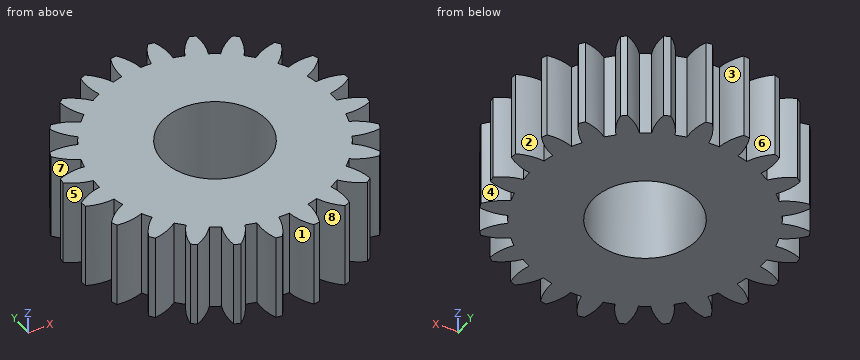
```python
from build123d import *

# Parameters (mm, degrees)
SKETCH2_R           = 3.81
BOSS_EXTRUDE1_DEPTH = 6.35


with BuildPart() as part:
    # Sketch2 → Boss-Extrude1 (new body)
    with BuildSketch(Plane.XY):
        with BuildLine():
            ThreePointArc((-42.015017319, -22.945367918), (-41.531469039, -22.120633406), (-41.268457962, -21.20148645))
            ThreePointArc((-41.268457962, -21.20148645), (-40.889005651, -21.209938725), (-40.50955334, -21.20148645))
            ThreePointArc((-40.50955334, -21.20148645), (-40.246542262, -22.120633406), (-39.762993983, -22.945367918))
            ThreePointArc((-39.762993983, -22.945367918), (-39.542138505, -22.918710388), (-39.321909019, -22.887297981))
            ThreePointArc((-39.321909019, -22.887297981), (-39.068294246, -21.965514112), (-39.052137791, -21.009614053))
            ThreePointArc((-39.052137791, -21.009614053), (-38.683427394, -20.919568839), (-38.319092217, -20.813195084))
            ThreePointArc((-38.319092217, -20.813195084), (-37.827150287, -21.632950591), (-37.146621516, -22.304431452))
            ThreePointArc((-37.146621516, -22.304431452), (-36.940190983, -22.221520651), (-36.735595764, -22.13417901))
            ThreePointArc((-36.735595764, -22.13417901), (-36.729197926, -21.178163832), (-36.960997129, -20.250653679))
            ThreePointArc((-36.960997129, -20.250653679), (-36.628155651, -20.068247408), (-36.303766447, -19.871201369))
            ThreePointArc((-36.303766447, -19.871201369), (-35.616418695, -20.535700443), (-34.785286345, -21.008167342))
            ThreePointArc((-34.785286345, -21.008167342), (-34.607348655, -20.874653505), (-34.432330529, -20.737334819))
            ThreePointArc((-34.432330529, -20.737334819), (-34.673585627, -19.812239186), (-35.137543756, -18.976327224))
            ThreePointArc((-35.137543756, -18.976327224), (-34.863253794, -18.713990582), (-34.600917152, -18.43970062))
            ThreePointArc((-34.600917152, -18.43970062), (-33.76500519, -18.903658748), (-32.839909556, -19.144913847))
            ThreePointArc((-32.839909556, -19.144913847), (-32.702590871, -18.969895721), (-32.569077034, -18.791958031))
            ThreePointArc((-32.569077034, -18.791958031), (-33.041543932, -17.960825681), (-33.706043007, -17.273477928))
            ThreePointArc((-33.706043007, -17.273477928), (-33.508996967, -16.949088725), (-33.326590697, -16.616247247))
            ThreePointArc((-33.326590697, -16.616247247), (-32.399080544, -16.84804645), (-31.443065365, -16.841648612))
            ThreePointArc((-31.443065365, -16.841648612), (-31.355723725, -16.637053393), (-31.272812924, -16.430622859))
            ThreePointArc((-31.272812924, -16.430622859), (-31.944293785, -15.750094089), (-32.764049292, -15.258152159))
            ThreePointArc((-32.764049292, -15.258152159), (-32.657675537, -14.893816982), (-32.567630323, -14.525106585))
            ThreePointArc((-32.567630323, -14.525106585), (-31.611730264, -14.50895013), (-30.689946395, -14.255335357))
            ThreePointArc((-30.689946395, -14.255335357), (-30.658533987, -14.035105871), (-30.631876458, -13.814250393))
            ThreePointArc((-30.631876458, -13.814250393), (-31.456610969, -13.330702114), (-32.375757925, -13.067691036))
            ThreePointArc((-32.375757925, -13.067691036), (-32.367305651, -12.688238725), (-32.375757925, -12.308786414))
            ThreePointArc((-32.375757925, -12.308786414), (-31.456610969, -12.045775337), (-30.631876458, -11.562227057))
            ThreePointArc((-30.631876458, -11.562227057), (-30.658533987, -11.341371579), (-30.689946395, -11.121142093))
            ThreePointArc((-30.689946395, -11.121142093), (-31.611730264, -10.86752732), (-32.567630323, -10.851370865))
            ThreePointArc((-32.567630323, -10.851370865), (-32.657675537, -10.482660468), (-32.764049292, -10.118325291))
            ThreePointArc((-32.764049292, -10.118325291), (-31.944293785, -9.626383361), (-31.272812924, -8.945854591))
            ThreePointArc((-31.272812924, -8.945854591), (-31.355723725, -8.739424057), (-31.443065365, -8.534828838))
            ThreePointArc((-31.443065365, -8.534828838), (-32.399080544, -8.528431), (-33.326590697, -8.760230203))
            ThreePointArc((-33.326590697, -8.760230203), (-33.508996967, -8.427388725), (-33.706043007, -8.102999522))
            ThreePointArc((-33.706043007, -8.102999522), (-33.041543932, -7.415651769), (-32.569077034, -6.584519419))
            ThreePointArc((-32.569077034, -6.584519419), (-32.702590871, -6.406581729), (-32.839909556, -6.231563603))
            ThreePointArc((-32.839909556, -6.231563603), (-33.76500519, -6.472818702), (-34.600917152, -6.936776831))
            ThreePointArc((-34.600917152, -6.936776831), (-34.863253794, -6.662486868), (-35.137543756, -6.400150226))
            ThreePointArc((-35.137543756, -6.400150226), (-34.673585627, -5.564238264), (-34.432330529, -4.639142631))
            ThreePointArc((-34.432330529, -4.639142631), (-34.607348655, -4.501823945), (-34.785286345, -4.368310108))
            ThreePointArc((-34.785286345, -4.368310108), (-35.616418695, -4.840777007), (-36.303766447, -5.505276082))
            ThreePointArc((-36.303766447, -5.505276082), (-36.628155651, -5.308230042), (-36.960997129, -5.125823771))
            ThreePointArc((-36.960997129, -5.125823771), (-36.729197926, -4.198313618), (-36.735595764, -3.24229844))
            ThreePointArc((-36.735595764, -3.24229844), (-36.940190983, -3.154956799), (-37.146621516, -3.072045999))
            ThreePointArc((-37.146621516, -3.072045999), (-37.827150287, -3.743526859), (-38.319092217, -4.563282366))
            ThreePointArc((-38.319092217, -4.563282366), (-38.683427394, -4.456908611), (-39.052137791, -4.366863397))
            ThreePointArc((-39.052137791, -4.366863397), (-39.068294246, -3.410963338), (-39.321909019, -2.489179469))
            ThreePointArc((-39.321909019, -2.489179469), (-39.542138505, -2.457767062), (-39.762993983, -2.431109532))
            ThreePointArc((-39.762993983, -2.431109532), (-40.246542262, -3.255844044), (-40.50955334, -4.174991))
            ThreePointArc((-40.50955334, -4.174991), (-40.889005651, -4.166538725), (-41.268457962, -4.174991))
            ThreePointArc((-41.268457962, -4.174991), (-41.531469039, -3.255844044), (-42.015017319, -2.431109532))
            ThreePointArc((-42.015017319, -2.431109532), (-42.235872797, -2.457767062), (-42.456102283, -2.489179469))
            ThreePointArc((-42.456102283, -2.489179469), (-42.709717056, -3.410963338), (-42.725873511, -4.366863397))
            ThreePointArc((-42.725873511, -4.366863397), (-43.094583907, -4.456908611), (-43.458919085, -4.563282366))
            ThreePointArc((-43.458919085, -4.563282366), (-43.950861015, -3.743526859), (-44.631389785, -3.072045999))
            ThreePointArc((-44.631389785, -3.072045999), (-44.837820319, -3.154956799), (-45.042415538, -3.24229844))
            ThreePointArc((-45.042415538, -3.24229844), (-45.048813376, -4.198313618), (-44.817014173, -5.125823771))
            ThreePointArc((-44.817014173, -5.125823771), (-45.149855651, -5.308230042), (-45.474244854, -5.505276082))
            ThreePointArc((-45.474244854, -5.505276082), (-46.161592607, -4.840777007), (-46.992724957, -4.368310108))
            ThreePointArc((-46.992724957, -4.368310108), (-47.170662646, -4.501823945), (-47.345680772, -4.639142631))
            ThreePointArc((-47.345680772, -4.639142631), (-47.104425674, -5.564238264), (-46.640467545, -6.400150226))
            ThreePointArc((-46.640467545, -6.400150226), (-46.914757508, -6.662486868), (-47.177094149, -6.936776831))
            ThreePointArc((-47.177094149, -6.936776831), (-48.013006112, -6.472818702), (-48.938101745, -6.231563603))
            ThreePointArc((-48.938101745, -6.231563603), (-49.075420431, -6.406581729), (-49.208934268, -6.584519419))
            ThreePointArc((-49.208934268, -6.584519419), (-48.736467369, -7.415651769), (-48.071968294, -8.102999522))
            ThreePointArc((-48.071968294, -8.102999522), (-48.269014334, -8.427388725), (-48.451420605, -8.760230203))
            ThreePointArc((-48.451420605, -8.760230203), (-49.378930758, -8.528431), (-50.334945936, -8.534828838))
            ThreePointArc((-50.334945936, -8.534828838), (-50.422287577, -8.739424057), (-50.505198377, -8.945854591))
            ThreePointArc((-50.505198377, -8.945854591), (-49.833717517, -9.626383361), (-49.01396201, -10.118325291))
            ThreePointArc((-49.01396201, -10.118325291), (-49.120335765, -10.482660468), (-49.210380979, -10.851370865))
            ThreePointArc((-49.210380979, -10.851370865), (-50.166281038, -10.86752732), (-51.088064907, -11.121142093))
            ThreePointArc((-51.088064907, -11.121142093), (-51.119477314, -11.341371579), (-51.146134844, -11.562227057))
            ThreePointArc((-51.146134844, -11.562227057), (-50.321400332, -12.045775337), (-49.402253376, -12.308786414))
            ThreePointArc((-49.402253376, -12.308786414), (-49.410705651, -12.688238725), (-49.402253376, -13.067691036))
            ThreePointArc((-49.402253376, -13.067691036), (-50.321400332, -13.330702114), (-51.146134844, -13.814250393))
            ThreePointArc((-51.146134844, -13.814250393), (-51.119477314, -14.035105871), (-51.088064907, -14.255335357))
            ThreePointArc((-51.088064907, -14.255335357), (-50.166281038, -14.50895013), (-49.210380979, -14.525106585))
            ThreePointArc((-49.210380979, -14.525106585), (-49.120335765, -14.893816982), (-49.01396201, -15.258152159))
            ThreePointArc((-49.01396201, -15.258152159), (-49.833717517, -15.750094089), (-50.505198377, -16.430622859))
            ThreePointArc((-50.505198377, -16.430622859), (-50.422287577, -16.637053393), (-50.334945936, -16.841648612))
            ThreePointArc((-50.334945936, -16.841648612), (-49.378930758, -16.84804645), (-48.451420605, -16.616247247))
            ThreePointArc((-48.451420605, -16.616247247), (-48.269014334, -16.949088725), (-48.071968294, -17.273477928))
            ThreePointArc((-48.071968294, -17.273477928), (-48.736467369, -17.960825681), (-49.208934268, -18.791958031))
            ThreePointArc((-49.208934268, -18.791958031), (-49.075420431, -18.969895721), (-48.938101745, -19.144913847))
            ThreePointArc((-48.938101745, -19.144913847), (-48.013006112, -18.903658748), (-47.177094149, -18.43970062))
            ThreePointArc((-47.177094149, -18.43970062), (-46.914757508, -18.713990582), (-46.640467545, -18.976327224))
            ThreePointArc((-46.640467545, -18.976327224), (-47.104425674, -19.812239186), (-47.345680772, -20.737334819))
            ThreePointArc((-47.345680772, -20.737334819), (-47.170662646, -20.874653505), (-46.992724957, -21.008167342))
            ThreePointArc((-46.992724957, -21.008167342), (-46.161592607, -20.535700443), (-45.474244854, -19.871201369))
            ThreePointArc((-45.474244854, -19.871201369), (-45.149855651, -20.068247408), (-44.817014173, -20.250653679))
            ThreePointArc((-44.817014173, -20.250653679), (-45.048813376, -21.178163832), (-45.042415538, -22.13417901))
            ThreePointArc((-45.042415538, -22.13417901), (-44.837820319, -22.221520651), (-44.631389785, -22.304431452))
            ThreePointArc((-44.631389785, -22.304431452), (-43.950861015, -21.632950591), (-43.458919085, -20.813195084))
            ThreePointArc((-43.458919085, -20.813195084), (-43.094583907, -20.919568839), (-42.725873511, -21.009614053))
            ThreePointArc((-42.725873511, -21.009614053), (-42.709717056, -21.965514112), (-42.456102283, -22.887297981))
            ThreePointArc((-42.456102283, -22.887297981), (-42.235872797, -22.918710388), (-42.015017319, -22.945367918))
        make_face()
        with Locations((-40.889005651, -12.688238725)):
            Circle(SKETCH2_R, mode=Mode.SUBTRACT)
    extrude(amount=BOSS_EXTRUDE1_DEPTH)


solid = part.part
```
Design review of the part built by this model. Coordinates are the model's own, in mm. Face numbers are marked on the shaded views. A direction names the side the tool comes from. Give positions to 0.01 mm unless a question says otherwise; leave off trailing zeros. Order: outer loops, then holes, each group sorted by start corner. A loop starts at its lowest first (then second) coordinate and runs counter-clockwise, first axis right, second up. Notation, with made-up numbers: (46.25, 51.5) -> (62.25, 51.5) arc R8 cw to (62.25, 60.5) -> close; hole circle Ø9 at (27, 79.25). An arc over 180 degrees is marked (long way). Write each question's results on one line, items separated by ' | '. Start each with the question number.
Q1. Add section C-C on y = -16. Give the boundary of the cut face in (x, z), and give its area (3 significant figures).
Q2. Add section B-B on x = -38. Give the boundary of the cut face in (y, z).
Q3. For pin 1 (3 mm diameter, centred on y = -19.5, z = 3, fed in from -X); pin 2 (2 mm diameter, centred on x = -37, z = 5.5, fed in from +Y); pin 3 (1.5 mm diameter, centred on x = -36.5, z = 3, fed in from -Y), all flat-tipped, find the tip position at first contact; note any pin that passes through.
Q4. Mouldability with a two-part tool opening along Y and no side actions: class the marked faces 5, 6, 7 and 8 as +Y half, -Y half, draft (parallel to the pull), parting line (faces both ways), or undercut.
Q5. Add section D-D on x = -46.25. Give the boundary of the cut face in (y, z), and give its area (3 significant figures).
Q6. Wall thickness on L1, parallel to X at y = -12.5, z = 2; L2, parallel to X at y = -3.75, z = 5.75; L3, parallel to Y at x = -48.75, z = 1: over which ranges is each line inside the solid? List them lowest first. Write a range as from..to.
Q7. Machinability: for the marked faces 1, 2, 3 and 4, which of the approach directions +Z, -Z, +X, -X, +Y, -Y give a long, thin tool a straight path to every point of the face, cutting with its end or side? Answer none if there is none.
Q8. Add section A-A on y = -21.5. Give the boundary of the cut face in (x, z).
Found:
1) outline: (-50.12, 0) -> (-42.77, 0) -> (-42.77, 6.35) -> (-50.12, 6.35) -> close; (-39.01, 0) -> (-31.66, 0) -> (-31.66, 6.35) -> (-39.01, 6.35) -> close | area: 93.3 mm2
2) outline: (-21.39, 0) -> (-15.17, 0) -> (-15.17, 6.35) -> (-21.39, 6.35) -> close; (-10.2, 0) -> (-3.98, 0) -> (-3.98, 6.35) -> (-10.2, 6.35) -> close
3) pin 1: stops at x = -49.21 | pin 2: stops at y = -3.07 | pin 3: stops at y = -22.3
4) face 5: undercut | face 6: +Y half | face 7: undercut | face 8: -Y half
5) outline: (-20.6, 0) -> (-4.78, 0) -> (-4.78, 6.35) -> (-20.6, 6.35) -> close | area: 100 mm2
6) L1: x = -49.41..-44.69, -37.08..-32.37 | L2: x = -45.08..-43.95, -42.74..-41.36, -40.42..-39.03, -37.83..-36.7 | L3: y = -19.12..-17.98, -16.72..-8.66, -7.4..-6.26
7) face 1: +Z, -Z, -Y | face 2: +Z, -Z | face 3: +Z, -Z, +Y | face 4: +Z, -Z, +X
8) outline: (-45.07, 0) -> (-43.85, 0) -> (-43.85, 6.35) -> (-45.07, 6.35) -> close; (-42.75, 0) -> (-41.33, 0) -> (-41.33, 6.35) -> (-42.75, 6.35) -> close; (-40.45, 0) -> (-39.03, 0) -> (-39.03, 6.35) -> (-40.45, 6.35) -> close; (-37.93, 0) -> (-36.7, 0) -> (-36.7, 6.35) -> (-37.93, 6.35) -> close
